from build123d import *

# Parameters (mm, degrees)
EXTRUDE_1_DEPTH      = 6
SKETCH_2_R           = 18.5
CUT_EXTRUDE_1_DEPTH  = 5
CHAMFER_1_SIZE       = 1.640243073
CHAMFER_1_SIZE_2     = 0.8
SKETCH_18_W          = 40
SKETCH_18_H          = 25
CUT_EXTRUDE_9_DEPTH  = 1
SKETCH_19_R          = 1.4
CUT_EXTRUDE_10_DEPTH = 152.410039297
SKETCH_20_R          = 2.25
CUT_EXTRUDE_11_DEPTH = 0.7
SKETCH_21_W          = 4
SKETCH_21_H          = 30
CUT_EXTRUDE_12_DEPTH = 152.446360141
SKETCH_22_R          = 1
CUT_EXTRUDE_13_DEPTH = 6
CUT_EXTRUDE_START    = -6
SKETCH_23_R          = 1
CUT_EXTRUDE_14_DEPTH = 6
SKETCH_24_R          = 17.5
CUT_EXTRUDE_15_DEPTH = 152.410039297


with BuildPart() as part:
    # 스케치1 → 보스-돌출1 (new body)
    with BuildSketch(Plane.XY):
        with BuildLine():
            Line((-20, 0), (-20, 130))
            ThreePointArc((-20, 130), (0, 150), (20, 130))
            Line((20, 130), (20, 0))
            ThreePointArc((20, 0), (0, -20), (-20, 0))
        make_face()
    extrude(amount=EXTRUDE_1_DEPTH)

    # 스케치2 → 컷-돌출1 (cut)
    with BuildSketch(Plane(origin=(0, 0, 0), x_dir=(-1, 0, 0), z_dir=(0, 0, -1))):
        Circle(SKETCH_2_R)
        with Locations((0, 130)):
            Circle(SKETCH_2_R)
    extrude(amount=-CUT_EXTRUDE_1_DEPTH, mode=Mode.SUBTRACT)

    # 모따기1
    # the kernel refuses this chamfer: 1.640243073, 0.8 mm, written as the material it takes off along each edge
    with BuildSketch(Plane(origin=(0, 130, 0), x_dir=(-1, 0, 0), z_dir=(0, -1, 0))) as chamfer_1_piece_1:
        Polygon((18.5 + CHAMFER_1_SIZE, 0), (18.5, -CHAMFER_1_SIZE_2), (18.5, 0), align=None)
    revolve(axis=Axis((0, 130, 0), (0, 0, -1)), mode=Mode.SUBTRACT)
    with BuildSketch(Plane(origin=(0, 0, 0), x_dir=(-1, 0, 0), z_dir=(0, -1, 0))) as chamfer_1_piece_2:
        Polygon((18.5 + CHAMFER_1_SIZE, 0), (18.5, -CHAMFER_1_SIZE_2), (18.5, 0), align=None)
    revolve(axis=Axis((0, 0, 0), (0, 0, -1)), mode=Mode.SUBTRACT)

    # 스케치18 → 컷-돌출9 (cut)
    with BuildSketch(Plane.XY.offset(6)):
        with Locations((0, 65)):
            Rectangle(SKETCH_18_W, SKETCH_18_H)
    extrude(amount=-CUT_EXTRUDE_9_DEPTH, mode=Mode.SUBTRACT)

    # 스케치19 → 컷-돌출10 (cut, through all)
    with BuildSketch(Plane.XY.offset(5)):
        with Locations((-12.5, 72.5)):
            Circle(SKETCH_19_R)
        with Locations((12.5, 72.5)):
            Circle(SKETCH_19_R)
        with Locations((-12.5, 57.5)):
            Circle(SKETCH_19_R)
        with Locations((12.5, 57.5)):
            Circle(SKETCH_19_R)
    extrude(amount=-CUT_EXTRUDE_10_DEPTH, mode=Mode.SUBTRACT)

    # 스케치20 → 컷-돌출11 (cut)
    with BuildSketch(Plane(origin=(0, 0, 0), x_dir=(-1, 0, 0), z_dir=(0, 0, -1))):
        with Locations((-12.5, 72.5)):
            Circle(SKETCH_20_R)
        with Locations((12.5, 72.5)):
            Circle(SKETCH_20_R)
        with Locations((-12.5, 57.5)):
            Circle(SKETCH_20_R)
        with Locations((12.5, 57.5)):
            Circle(SKETCH_20_R)
    extrude(amount=-CUT_EXTRUDE_11_DEPTH, mode=Mode.SUBTRACT)

    # 스케치21 → 컷-돌출12 (cut, through all)
    with BuildSketch(Plane.XY.offset(6)):
        with Locations((-20, 103.75)):
            Rectangle(SKETCH_21_W, SKETCH_21_H)
        with Locations((20, 103.75)):
            Rectangle(SKETCH_21_W, SKETCH_21_H)
        with Locations((-20, 26.25)):
            Rectangle(SKETCH_21_W, SKETCH_21_H)
        with Locations((20, 26.25)):
            Rectangle(SKETCH_21_W, SKETCH_21_H)
    extrude(amount=-CUT_EXTRUDE_12_DEPTH, mode=Mode.SUBTRACT)

    # 스케치22 → 컷-돌출13 (cut)
    with BuildSketch(Plane(origin=(18, 0, 0), x_dir=(0, 0, -1), z_dir=(1, 0, 0))):
        with Locations(Location((-3, 16.25, 0), (0, 0, 90))):
            Circle(SKETCH_22_R)
        with Locations(Location((-3, 36.25, 0), (0, 0, 90))):
            Circle(SKETCH_22_R)
        with Locations(Location((-3, 113.75, 0), (0, 0, 90))):
            Circle(SKETCH_22_R)
        with Locations(Location((-3, 93.75, 0), (0, 0, 90))):
            Circle(SKETCH_22_R)
    extrude(amount=-CUT_EXTRUDE_13_DEPTH, mode=Mode.SUBTRACT)

    # 스케치23 → 컷-돌출14 (cut)
    with BuildSketch(Plane.ZY.offset(18).offset(CUT_EXTRUDE_START)):
        with Locations(Location((3, 16.25, 0), (0, 0, 90))):
            Circle(SKETCH_23_R)
        with Locations(Location((3, 36.25, 0), (0, 0, 90))):
            Circle(SKETCH_23_R)
        with Locations(Location((3, 113.75, 0), (0, 0, 90))):
            Circle(SKETCH_23_R)
        with Locations(Location((3, 93.75, 0), (0, 0, 90))):
            Circle(SKETCH_23_R)
    extrude(amount=CUT_EXTRUDE_14_DEPTH, mode=Mode.SUBTRACT)

    # 스케치24 → 컷-돌출15 (cut, through all)
    with BuildSketch(Plane(origin=(0, 0, 5), x_dir=(-1, 0, 0), z_dir=(0, 0, -1))):
        with Locations((0, 130)):
            Circle(SKETCH_24_R)
        Circle(SKETCH_24_R)
    extrude(amount=-CUT_EXTRUDE_15_DEPTH, mode=Mode.SUBTRACT)


solid = part.part
Could you check a few things on this model? Use its own coordinates, in mm. A direction names the side the tool comes from. Coordinates: 2 decimals unless noted, no trailing zeros. Order: outer loops, then holes, each group sorted by start corner. A loop starts at its lowest first (then second) coordinate and runs counter-clockwise, first axis right, second up. Notation, with made-up numbers: (77, 82.25) -> (101, 82.25) arc R30 ccw to (101, 114.25) -> close; hole circle Ø7 at (31.5, 41). An arc over 180 degrees is marked (long way). One line per question, with ' | ' between items.
Q1. I'm going to push flat-ended pins straight in: P1, Ø1.6, axis at y = 36.5, z = 2.5, coming from the +X side; P2, Ø2, axis at x = -19.5, z = 2, coming from the +Y side; P3, Ø1.2, axis at y = 113.75, z = 3, coming from the -X side. Where does each tip first touch, or does it pass through?
Return value:
P1: x = 18 | P2: y = 137.6 | P3: x = -12
Q2. Thinking about a two-plate mould opening in Y: for faces 6 (the face through (0, 25, 6)), 7 (the face through (-13.61, 71.65, 2.88)), 8 (the face through (0, 150, 3)), which applies, pulls with the +Y half, pulls with the -Y half, needs draft (parallel to the pull), parting line crosses it, or undercut?
Return value:
face 6: needs draft | face 7: undercut | face 8: pulls with the +Y half
Q3. If I drill on L1, parallel to X at y = 72.5, z = 2.5; L2, parallel to Y at x = 3, z = 1.65; L3, parallel to Y at x = -13.5, z = 4.1, over which ranges is the centre line in solid material (lowest first)?
Return value:
L1: -20 to -13.9, -11.1 to 11.1, 13.9 to 20 | L2: -19.77 to -18.26, 18.26 to 111.74, 148.26 to 149.77 | L3: -14.76 to -12.65, 12.65 to 56.52, 58.48 to 71.52, 73.48 to 117.35, 142.65 to 144.76
Q4. On a 3-axis mill with a long thin cutter (end or side, diameter ignored), from which of +Z, -Z, +X, -X, +Y, -Y can I reach the whole of each face in a straight line? I mean faces 1 (the face through (12, 74, 0.7)), 2 (the face through (-20, 124, 3)), 3 (the face through (-18, 104, 3)), 4 (the face through (18, 26, 3)), 5 (the face through (20, 6, 3)). Say none if no direction works.
Return value:
face 1: -Z | face 2: +Z, -Z, -X, +Y, -Y | face 3: +Z, -Z, -X | face 4: +Z, -Z, +X | face 5: +Z, -Z, +X, +Y, -Y
Q5. Imagine slicing it at C-C on y = 108. Please give me the cut outline in (x, z).
Return value:
outline: (-18, 0) -> (18, 0) -> (18, 6) -> (-18, 6) -> close
Q6. Imagine slicing it at B-B on z = 3. State how many separate pieces and enclosed holes the cut face has, and give its area (3 significant figures).
Return value:
separate pieces: 1 | enclosed holes: 6 | area: 3,950 mm²
Q7. Imagine slicing it at A-A on y = 72.5. Please give me the cut outline in (x, z), and give its area (3 significant figures).
Return value:
outline: (-20, 0) -> (-14.75, 0) -> (-14.75, 0.7) -> (-13.9, 0.7) -> (-13.9, 5) -> (-20, 5) -> close; (-11.1, 0.7) -> (-10.25, 0.7) -> (-10.25, 0) -> (10.25, 0) -> (10.25, 0.7) -> (11.1, 0.7) -> (11.1, 5) -> (-11.1, 5) -> close; (13.9, 0.7) -> (14.75, 0.7) -> (14.75, 0) -> (20, 0) -> (20, 5) -> (13.9, 5) -> close | area: 170 mm²
